CAD build for the part. Positions are in the model's coordinates, mm. A direction names the side the tool comes from. Coordinates: 2 decimals unless noted, no trailing zeros. Use one line per item in the form item = value.
```python
from build123d import *

# Parameters (mm, degrees)
F0_R     = 3
F1_DEPTH = 3
F2_R     = 5
F3_R     = 5
F4_R     = 5
F5_R     = 5
F6_R     = 3.5
F7_R     = 3.5
F8_R     = 3.5
F9_R     = 3.5


with BuildPart() as f1:
    # F0 (on Top) → F1 (new body)
    with BuildSketch(Plane.XY):
        with BuildLine():
            ThreePointArc((73.665267, 27.584182), (74.664819, 32.497377), (75, 37.5))
            Line((75, 37.5), (56.3, 37.5))
            Line((56.3, 37.5), (69.082022, 57.719443))
            ThreePointArc((69.082022, 57.719443), (64.132536, 63.899962), (57.995666, 68.903466))
            Line((57.995666, 68.903466), (50.514808, 57.069753))
            Line((50.514808, 57.069753), (48.427588, 73.372522))
            ThreePointArc((48.427588, 73.372522), (43.024058, 74.590899), (37.5, 75))
            Line((37.5, 75), (37.5, 56.3))
            Line((37.5, 56.3), (16.751921, 68.737273))
            ThreePointArc((16.751921, 68.737273), (10.54359, 63.569176), (5.586086, 57.191421))
            Line((5.586086, 57.191421), (16.751921, 48.74606))
            Line((16.751921, 48.74606), (1.253953, 47.116346))
            ThreePointArc((1.253953, 47.116346), (0.31481, 42.348879), (0, 37.5))
            Line((0, 37.5), (18.7, 37.5))
            Line((18.7, 37.5), (6.938024, 15.769478))
            ThreePointArc((6.938024, 15.769478), (11.763487, 10.225802), (17.577552, 5.729793))
            Line((17.577552, 5.729793), (24.635362, 17.820587))
            Line((24.635362, 17.820587), (28.01219, 1.220096))
            ThreePointArc((28.01219, 1.220096), (32.717031, 0.306275), (37.5, 0))
            Line((37.5, 0), (37.5, 18.7))
            Line((37.5, 18.7), (58.640158, 6.526726))
            ThreePointArc((58.640158, 6.526726), (64.467307, 11.442096), (69.179969, 17.434369))
            Line((69.179969, 17.434369), (57.719454, 22.204241))
            Line((57.719454, 22.204241), (73.665267, 27.584182))
        make_face()
        with Locations((37.5, 37.5)):
            Circle(F0_R, mode=Mode.SUBTRACT)
    extrude(amount=F1_DEPTH)

    # F2
    f2_edges = [f1.edges().sort_by_distance(p)[0] for p in [
        (37.5, 18.7, 1.5),
    ]]
    fillet(f2_edges, radius=F2_R)

    # F3
    f3_edges = [f1.edges().sort_by_distance(p)[0] for p in [
        (56.3, 37.5, 1.5),
    ]]
    fillet(f3_edges, radius=F3_R)

    # F4
    f4_edges = [f1.edges().sort_by_distance(p)[0] for p in [
        (18.7, 37.5, 1.5),
    ]]
    fillet(f4_edges, radius=F4_R)

    # F5
    f5_edges = [f1.edges().sort_by_distance(p)[0] for p in [
        (37.5, 56.3, 1.5),
    ]]
    fillet(f5_edges, radius=F5_R)

    # F6
    f6_edges = [f1.edges().sort_by_distance(p)[0] for p in [
        (24.635362, 17.820587, 1.5),
    ]]
    fillet(f6_edges, radius=F6_R)

    # F7
    f7_edges = [f1.edges().sort_by_distance(p)[0] for p in [
        (57.719454, 22.204241, 1.5),
    ]]
    fillet(f7_edges, radius=F7_R)

    # F8
    f8_edges = [f1.edges().sort_by_distance(p)[0] for p in [
        (50.514808, 57.069753, 1.5),
    ]]
    fillet(f8_edges, radius=F8_R)

    # F9
    f9_edges = [f1.edges().sort_by_distance(p)[0] for p in [
        (16.751921, 48.74606, 1.5),
    ]]
    fillet(f9_edges, radius=F9_R)


solid = f1.part
```
Item 1: Drop flat-ended pins along their axis: pin 1 (0.9 mm diameter, centred on y = 69.5, z = 2, fed in from -X); pin 2 (5 mm diameter, centred on x = 67, y = 24, fed in from -Z); pin 3 (1 mm diameter, centred on y = 10.5, z = 1, fed in from +X); pin 4 (0.9 mm diameter, centred on y = 7, z = 1, fed in from +X). Give the stop position or say it passes through.
Derived:
pin_1 = 37.5
pin_2 = 0
pin_3 = 64.03
pin_4 = 59.93
Item 2: Two-plate mould, pull along Y, no slides. Class faces 1 (the face through (52.05, 63.73, 1.52)), 2 (the face through (64.393, 11.365, 1.479)), 3 (the face through (64.152, 21.923, 1.521)): +Y half, -Y half, draft (parallel to the pull), parting line (faces both ways), or undercut.
Derived:
face_1 = +Y half
face_2 = -Y half
face_3 = undercut
Item 3: Drill centre lines: line 1 (Y direction, x = 9.5, z = 0.8); line 2 (Y direction, x = 70, z = 1.2); line 3 (X direction, y = 16.5, z = 2.9). Where is each one in solid material? Low to high. Write a range as [from, to].
Derived:
line_1 = [12.56, 20.5], [37.5, 48.38], [54.23, 62.44]
line_2 = [26.35, 37.5]
line_3 = [7.33, 68.57]
Item 4: 3-axis set-ups, long thin cutter, end or side, ignore diameter. For faces 4 (the face through (4.643, 47.473, 1.479)), 5 (the face through (48.86, 70, 1.48)), 6 (the face through (51.72, 10.51, 1.48)): which of +Z, -Z, +X, -X, +Y, -Y reach the whole face in a straight line?
Derived:
face_4 = +Z, -Z, -X
face_5 = +Z, -Z, +Y
face_6 = +Z, -Z, -Y
